from build123d import *

# Parameters (mm, degrees)
BOSS_EXTRU_1_DEPTH = 21
BOSS_EXTRU_2_DEPTH = 3
BOSS_EXTRU_3_START = 3
BOSS_EXTRU_3_DEPTH = 3
BOSS_EXTRU_5_START = 3
BOSS_EXTRU_5_DEPTH = 3


with BuildPart() as part:
    # Esquisse1 → Boss.-Extru.1 (new body)
    with BuildSketch(Plane(origin=(0, 0, 0), x_dir=(1, 0, 0), z_dir=(0, 1, 0))):
        with BuildLine():
            ThreePointArc((-19.357142857, 1.428571429), (-3.857142857, 16.928571429), (11.642857143, 1.428571429))
            Line((11.642857143, 1.428571429), (21.642857143, 1.428571429))
            Line((21.642857143, 1.428571429), (21.642857143, -9.071428571))
            Line((21.642857143, -9.071428571), (11.642857143, -9.071428571))
            Line((11.642857143, -9.071428571), (6.642857143, -9.071428571))
            Line((6.642857143, -9.071428571), (6.642857143, 1.428571429))
            ThreePointArc((6.642857143, 1.428571429), (-3.857142857, 11.928571429), (-14.357142857, 1.428571429))
            Line((-14.357142857, 1.428571429), (-14.357142857, -9.071428571))
            Line((-14.357142857, -9.071428571), (-19.357142857, -9.071428571))
            Line((-19.357142857, -9.071428571), (-29.357142857, -9.071428571))
            Line((-29.357142857, -9.071428571), (-29.357142857, 1.428571429))
            Line((-29.357142857, 1.428571429), (-19.357142857, 1.428571429))
        make_face()
    extrude(amount=BOSS_EXTRU_1_DEPTH)

    # Esquisse2 → Boss.-Extru.2 (add)
    with BuildSketch(Plane(origin=(0, 21, 0), x_dir=(1, 0, 0), z_dir=(0, 1, 0))):
        with BuildLine():
            Line((-18.148749115, 7.428571429), (-10.148749115, 7.428571429))
            ThreePointArc((-10.148749115, 7.428571429), (-3.857142857, 10.122495129), (2.4344634, 7.428571429))
            Line((2.4344634, 7.428571429), (10.4344634, 7.428571429))
            ThreePointArc((10.4344634, 7.428571429), (-3.857142857, 16.928571733), (-18.148749115, 7.428571429))
        make_face()
    extrude(amount=BOSS_EXTRU_2_DEPTH)

    # Esquisse3 → Boss.-Extru.3 (add)
    with BuildSketch(Plane(origin=(0, 0, 0), x_dir=(-1, 0, 0), z_dir=(0, -1, 0)).offset(BOSS_EXTRU_3_START)):
        with BuildLine():
            Line((-10.434463071, 7.428571429), (-2.434463071, 7.428571429))
            ThreePointArc((-2.434463071, 7.428571429), (3.857142857, 10.12249489), (10.148748785, 7.428571429))
            Line((10.148748785, 7.428571429), (18.148748785, 7.428571429))
            ThreePointArc((18.148748785, 7.428571429), (3.857142857, 16.928571429), (-10.434463071, 7.428571429))
        make_face()
    extrude(amount=-BOSS_EXTRU_3_DEPTH)

    # Esquisse5 → Boss.-Extru.5 (add)
    with BuildSketch(Plane.XZ.offset(BOSS_EXTRU_5_START)):
        with BuildLine():
            Line((-18.148748785, -7.428571429), (-12.473986827, -7.428571429))
            ThreePointArc((-12.473986827, -7.428571429), (-13.875297919, -4.572862948), (-14.357142857, -1.428571429))
            Line((-14.357142857, -1.428571429), (-14.357142857, 9.071428571))
            Line((-14.357142857, 9.071428571), (-29.357142857, 9.071428571))
            Line((-29.357142857, 9.071428571), (-29.357142857, -1.428571429))
            Line((-29.357142857, -1.428571429), (-19.357142857, -1.428571429))
            ThreePointArc((-19.357142857, -1.428571429), (-19.052041539, -4.488809011), (-18.148748785, -7.428571429))
        make_face()
        with BuildLine():
            Line((4.759701113, -7.428571429), (10.434463071, -7.428571429))
            ThreePointArc((10.434463071, -7.428571429), (11.337755824, -4.488809011), (11.642857143, -1.428571429))
            Line((11.642857143, -1.428571429), (21.642857143, -1.428571429))
            Line((21.642857143, -1.428571429), (21.642857143, 9.071428571))
            Line((21.642857143, 9.071428571), (6.642857143, 9.071428571))
            Line((6.642857143, 9.071428571), (6.642857143, -1.428571429))
            ThreePointArc((6.642857143, -1.428571429), (6.161012205, -4.572862948), (4.759701113, -7.428571429))
        make_face()
    extrude(amount=-BOSS_EXTRU_5_DEPTH)


solid = part.part
Geometry check sheet. Reference: the model listing, model coordinates, mm. A direction names the side the tool comes from. Round coordinates to 2 decimals unless told otherwise and drop trailing zeros. Write each loop counter-clockwise with the first axis right and the second up, starting at its lowest first coordinate (ties: lowest second). Pieces come first, ordered by that corner, then holes. Notation, with made-up numbers: (-31, 16.25) - (-5, 16.25) arc R19 cw to (-5, 32.25) - close; hole circle Ø8 at (54, 16). An arc over 180 degrees is marked (long way). One line per item, written item: value.
1. Cross-section at D-D on z = -11. Record the boundary of the cut face in (x, y), and give its area (3 significant figures).
The answers:
outline: (-16.05, -3) - (8.33, -3) - (8.33, 24) - (-16.05, 24) - close; hole (-8.17, 0) - (0.46, 0) - (0.46, 21) - (-8.17, 21) - close
area: 477 mm^2
2. Cross-section at C-C on x = 13. Record the boundary of the cut face in (y, z).
The answers:
outline: (-3, -1.43) - (21, -1.43) - (21, 9.07) - (-3, 9.07) - close
3. Cross-section at B-B on y = 14.25. Record the boundary of the cut face in (x, z).
The answers:
outline: (-29.36, -1.43) - (-19.36, -1.43) arc R15.5 ccw to (11.64, -1.43) - (21.64, -1.43) - (21.64, 9.07) - (6.64, 9.07) - (6.64, -1.43) arc R10.5 cw to (-14.36, -1.43) - (-14.36, 9.07) - (-29.36, 9.07) - close
4. Scan lines: L1, parallel to X at y = 2, z = 7.5; L2, parallel to Y at x = -24.5, z = 1; L3, parallel to X at y = 5.5, z = -5.25. Record each from-to range of solid material in increasing order.
The answers:
L1: x = -29.36 to -14.36, 6.64 to 21.64
L2: y = -3 to 21
L3: x = -18.88 to -13.64, 5.92 to 11.16
5. Cross-section at A-A on z = 3. Record the boundary of the cut face in (x, y), and give its area (3 significant figures).
The answers:
outline: (-29.36, -3) - (-14.36, -3) - (-14.36, 21) - (-29.36, 21) - close; (6.64, -3) - (21.64, -3) - (21.64, 21) - (6.64, 21) - close
area: 720 mm^2
6. Set-up check for faces 1 (the face through (-21, 21, 3)), 2 (the face through (-4, 21, -11)), 3 (the face through (4, -2, -7.429)), 4 (the face through (17, 9, -1.429)), 5 (the face through (-24, 9, -1.429)): record each of +Z, -Z, +X, -X, +Y, -Y from which the full face is reachable in a straight line by a thin tool's end or side.
The answers:
face 1: +Z, +X, -X, +Y
face 2: +Z
face 3: +Z, +Y, -Y
face 4: -Z, +X, +Y, -Y
face 5: -Z, -X, +Y, -Y
7. Depth check by flat-ended pin: pin 1 Ø12 at (y, z) = (20, -10) entering from +X; pin 2 Ø3 at (x, y) = (-19.5, 12.5) entering from -Z; pin 3 Ø1.2 at (x, y) = (4, -2) entering from +Z. Enter the tip coordinate at first touch or a pass-through.
The answers:
pin 1: stops at x = 11.43
pin 2: stops at z = -7.77
pin 3: stops at z = -7.43
